Geometry: final body of the model. Coordinates: model frame, mm. Face numbers are marked on the shaded views. Give positions to 0.01 mm unless a question says otherwise; leave off trailing zeros. Write each loop counter-clockwise with the first axis right and the second up, starting at its lowest first coordinate (ties: lowest second). Pieces come first, ordered by that corner, then holes. Notation, with made-up numbers: M 67.5,21 L 79.5,21 A11 cw 79.5,39 Z; hole C 54,-6.5 d11. An arc over 180 degrees is marked long. Use a Markdown table: item, result. Add a question column.
(1) Cut plane B-B (x = 3). Output: boundary loops of the cut face in (y, z), plus the area to 3 significant figures.
(2) Draft query along Z for the marked faces 1, 2 and 3. Return one class per face: released by +Z, released by -Z, zero draft, split by the parting line, or undercut.
(3) Cut plane D-D (x = -18). Output: boundary loops of the cut face in (y, z), plus the area to 3 significant figures.
(4) Cut plane A-A (y = 10). Output: boundary loops of the cut face in (x, z), plus the area to 3 significant figures.
(5) Pin query (flat end, axial travel): pin 1 Ø1 at (x, z) = (-34.5, 7.5) entering from +Y; pin 2 Ø1.6 at (x, z) = (-56, 31) entering from +Y; pin 3 Ø5.5 at (x, z) = (-27.5, -27.5) entering from -Y. Return the tip coordinate at first contact, or that it passes through.
(6) Cut plane C-C (z = -9.5). Output: boundary loops of the cut face in (x, y), plus the area to 4 significant figures.
(7) Material intervals for L1, parallel to X at y = -0.1, z = 24; L2, parallel to X at y = 46.25, z = 31; L3, parallel to Z at x = 53, y = -1, sorted ascending.
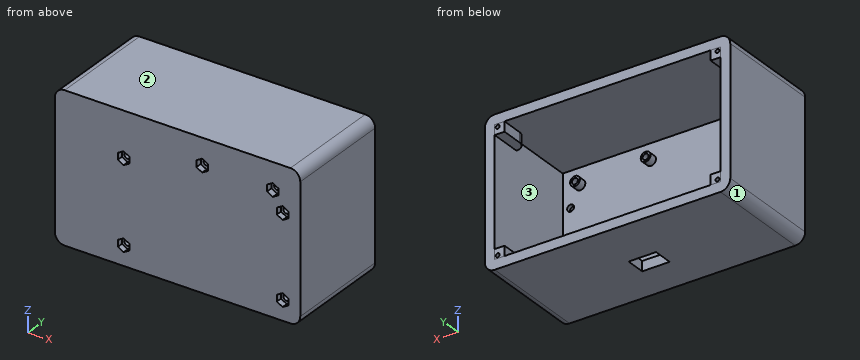
```python
from build123d import *

# Parameters (mm, degrees)
CROQUIS1_W                        = 125
CROQUIS1_H                        = 75
CROQUIS1_W_2                      = 115
CROQUIS1_H_2                      = 65
SALIENTE_EXTRUIR1_DEPTH           = 50
CROQUIS2_W                        = 125
CROQUIS2_H                        = 75
SALIENTE_EXTRUIR2_DEPTH           = 5
REDONDEO1_R                       = 5
SALIENTE_EXTRUIR3_DEPTH           = 10
CORTAR_EXTRUIR1_DEPTH             = 8
CROQUIS6_R                        = 1.75
CORTAR_EXTRUIR4_DEPTH             = 2
CORTAR_EXTRUIR5_DEPTH             = 5
SALIENTE_EXTRUIR4_DEPTH           = 0.001
SALIENTE_EXTRUIR4_DEPTH_BACK      = 16
CROQUIS8_W                        = 5
CROQUIS8_H                        = 5
REDONDEO2_R                       = 5
DI_METRO_DE_TALADRO_2_0_2_4_D     = 2
DI_METRO_DE_TALADRO_2_0_2_4_DEPTH = 10
DI_METRO_DE_TALADRO_2_0_2_4_TIP   = 0.600860619
CROQUIS11_R                       = 2.5
SALIENTE_EXTRUIR5_DEPTH           = 4
CROQUIS13_R                       = 1.5
CORTAR_EXTRUIR6_DEPTH             = 9
CORTAR_EXTRUIR7_DEPTH             = 3.2


with BuildPart() as part:
    # Croquis1 → Saliente-Extruir1 (new body)
    with BuildSketch(Plane(origin=(0, 0, 0), x_dir=(1, 0, 0), z_dir=(0, 1, 0))):
        Rectangle(CROQUIS1_W, CROQUIS1_H)
        Rectangle(CROQUIS1_W_2, CROQUIS1_H_2, mode=Mode.SUBTRACT)
    extrude(amount=SALIENTE_EXTRUIR1_DEPTH)

    # Croquis2 → Saliente-Extruir2 (add)
    with BuildSketch(Plane.XZ):
        Rectangle(CROQUIS2_W, CROQUIS2_H)
    extrude(amount=SALIENTE_EXTRUIR2_DEPTH)

    # Redondeo1
    redondeo1_edges = [part.edges().sort_by_distance(p)[0] for p in [
        (62.5, 22.5, 37.5),
        (-62.5, 22.5, 37.5),
        (-62.5, 22.5, -37.5),
        (62.5, 22.5, -37.5),
    ]]
    fillet(redondeo1_edges, radius=REDONDEO1_R)

    # Croquis3 → Saliente-Extruir3 (add)
    with BuildSketch(Plane(origin=(0, 0, 0), x_dir=(1, 0, 0), z_dir=(0, 1, 0))):
        Polygon((53.5, 24.151368439), (56.4, 25.825684219), (56.4, 29.174315781), (53.5, 30.848631561), (50.6, 29.174315781), (50.6, 25.825684219), align=None)
        Polygon((-24.6, 25.825684219), (-27.5, 24.151368439), (-30.4, 25.825684219), (-30.4, 29.174315781), (-27.5, 30.848631561), (-24.6, 29.174315781), align=None)
        Polygon((-24.6, -16.174315781), (-24.6, -12.825684219), (-27.5, -11.151368439), (-30.4, -12.825684219), (-30.4, -16.174315781), (-27.5, -17.848631561), align=None)
        Polygon((50.6, -12.825684219), (53.5, -11.151368439), (56.4, -12.825684219), (56.4, -16.174315781), (53.5, -17.848631561), (50.6, -16.174315781), align=None)
    extrude(amount=-SALIENTE_EXTRUIR3_DEPTH)

    # Croquis4 → Cortar-Extruir1 (cut)
    with BuildSketch(Plane.XZ.offset(10)):
        Polygon((53.5, -24.151368439), (50.6, -25.825684219), (50.6, -29.174315781), (53.5, -30.848631561), (56.4, -29.174315781), (56.4, -25.825684219), align=None)
        Polygon((50.6, 16.174315781), (50.6, 12.825684219), (53.5, 11.151368439), (56.4, 12.825684219), (56.4, 16.174315781), (53.5, 17.848631561), align=None)
        Polygon((-24.6, 16.174315781), (-27.5, 17.848631561), (-30.4, 16.174315781), (-30.4, 12.825684219), (-27.5, 11.151368439), (-24.6, 12.825684219), align=None)
        Polygon((-24.6, -29.174315781), (-24.6, -25.825684219), (-27.5, -24.151368439), (-30.4, -25.825684219), (-30.4, -29.174315781), (-27.5, -30.848631561), align=None)
    extrude(amount=-CORTAR_EXTRUIR1_DEPTH, mode=Mode.SUBTRACT)

    # Croquis6 → Cortar-Extruir4 (cut)
    with BuildSketch(Plane.XZ.offset(2)):
        with Locations(Location((53.5, -27.5, 0), (0, 0, 270))):
            Circle(CROQUIS6_R)
        with Locations(Location((-27.5, -27.5, 0), (0, 0, 270))):
            Circle(CROQUIS6_R)
        with Locations(Location((-27.5, 14.5, 0), (0, 0, 270))):
            Circle(CROQUIS6_R)
        with Locations(Location((53.5, 14.5, 0), (0, 0, 270))):
            Circle(CROQUIS6_R)
    extrude(amount=-CORTAR_EXTRUIR4_DEPTH, mode=Mode.SUBTRACT)

    # Croquis7 → Cortar-Extruir5 (cut)
    with BuildSketch(Plane.XY.offset(-32.5)):
        Polygon((-3.928571429, 23.75), (7.5, 23.75), (7.5, 13.75), (-5.131578947, 13.75), (-6.5, 13.75), (-6.5, 23.75), align=None)
    extrude(amount=-CORTAR_EXTRUIR5_DEPTH, mode=Mode.SUBTRACT)

    # Croquis8 → Saliente-Extruir4 (add, two sides: drawn at the far end of the back side and taken through both)
    with BuildSketch(Plane(origin=(0, 50, 0), x_dir=(1, 0, 0), z_dir=(0, 1, 0)).offset(-SALIENTE_EXTRUIR4_DEPTH_BACK)):
        with Locations((-55, -30)):
            Rectangle(CROQUIS8_W, CROQUIS8_H)
        with Locations((55, -30)):
            Rectangle(CROQUIS8_W, CROQUIS8_H)
        with Locations((55, 30)):
            Rectangle(CROQUIS8_W, CROQUIS8_H)
        with Locations((-55, 30)):
            Rectangle(CROQUIS8_W, CROQUIS8_H)
    extrude(amount=SALIENTE_EXTRUIR4_DEPTH + SALIENTE_EXTRUIR4_DEPTH_BACK)

    # Redondeo2
    redondeo2_edges = [part.edges().sort_by_distance(p)[0] for p in [
        (-52.5, 34, -30),
        (-52.5, 34, 30),
        (52.5, 34, 30),
        (52.5, 34, -30),
    ]]
    fillet(redondeo2_edges, radius=REDONDEO2_R - 0.0001)  # a hair under: the kernel refuses the full size

    # Diámetro de taladro Ø2.0 (2)4
    with Locations(Plane(origin=(-56, 50.001, -31), x_dir=(0, 0, 1), z_dir=(0, 1, 0))):
        with Locations((0, 0), (0, 112), (62, 112), (62, 0)):
            Hole(DI_METRO_DE_TALADRO_2_0_2_4_D / 2, depth=DI_METRO_DE_TALADRO_2_0_2_4_DEPTH)
            with Locations((0, 0, -(DI_METRO_DE_TALADRO_2_0_2_4_DEPTH + DI_METRO_DE_TALADRO_2_0_2_4_TIP / 2))):  # 118° drill point
                Cone(0, DI_METRO_DE_TALADRO_2_0_2_4_D / 2, DI_METRO_DE_TALADRO_2_0_2_4_TIP, mode=Mode.SUBTRACT)

    # Croquis11 → Saliente-Extruir5 (add)
    with BuildSketch(Plane(origin=(0, 0, 0), x_dir=(1, 0, 0), z_dir=(0, 1, 0))):
        with Locations(Location((12.5, -24, 0), (0, 0, 270))):
            Circle(CROQUIS11_R)
        with Locations(Location((48.5, -24, 0), (0, 0, 270))):
            Circle(CROQUIS11_R)
    extrude(amount=SALIENTE_EXTRUIR5_DEPTH)

    # Croquis13 → Cortar-Extruir6 (cut)
    with BuildSketch(Plane(origin=(0, 4, 0), x_dir=(1, 0, 0), z_dir=(0, 1, 0))):
        with Locations(Location((12.5, -24, 0), (0, 0, 270))):
            Circle(CROQUIS13_R)
        with Locations(Location((48.5, -24, 0), (0, 0, 270))):
            Circle(CROQUIS13_R)
    extrude(amount=-CORTAR_EXTRUIR6_DEPTH, mode=Mode.SUBTRACT)

    # Croquis14 → Cortar-Extruir7 (cut)
    with BuildSketch(Plane.XZ.offset(5)):
        Polygon((12.5, 20.651368439), (15.4, 22.325684219), (15.4, 25.674315781), (12.5, 27.348631561), (9.6, 25.674315781), (9.6, 22.325684219), align=None)
        Polygon((48.5, 20.651368439), (51.4, 22.325684219), (51.4, 25.674315781), (48.5, 27.348631561), (45.6, 25.674315781), (45.6, 22.325684219), align=None)
    extrude(amount=-CORTAR_EXTRUIR7_DEPTH, mode=Mode.SUBTRACT)


solid = part.part
```
Answer list:
| question | item | result |
|---|---|---|
| 1 | outline | M -5,-37.5 L 13.75,-37.5 L 13.75,-32.5 L 0,-32.5 L 0,32.5 L 50,32.5 L 50,37.5 L -5,37.5 Z; M 23.75,-37.5 L 50,-37.5 L 50,-32.5 L 23.75,-32.5 Z |
| 1 | area | 825 mm² |
| 2 | face 1 | released by -Z |
| 2 | face 2 | released by +Z |
| 2 | face 3 | undercut |
| 3 | outline | M -5,-37.5 L 50,-37.5 L 50,-32.5 L 0,-32.5 L 0,32.5 L 50,32.5 L 50,37.5 L -5,37.5 Z |
| 3 | area | 875 mm² |
| 4 | outline | M -62.5,-32.5 A5 ccw -57.5,-37.5 L 57.5,-37.5 A5 ccw 62.5,-32.5 L 62.5,32.5 A5 ccw 57.5,37.5 L -57.5,37.5 A5 ccw -62.5,32.5 Z; hole M -57.5,-32.5 L 57.5,-32.5 L 57.5,32.5 L -57.5,32.5 Z |
| 4 | area | 1,880 mm² |
| 5 | pin 1 | y = 0 |
| 5 | pin 2 | y = 39.88 |
| 5 | pin 3 | y = -2 |
| 6 | outline | M -62.5,-5 L 62.5,-5 L 62.5,50 L 57.5,50 L 57.5,0 L -57.5,0 L -57.5,50 L -62.5,50 Z |
| 6 | area | 1,125 mm² |
| 7 | L1 | -62.5 to 11, 14 to 47, 50 to 62.5 |
| 7 | L2 | -62.5 to -57, -55 to -52.5, 52.5 to 55, 57 to 62.5 |
| 7 | L3 | -37.5 to -29.18, -25.82 to 12.82, 16.18 to 37.5 |
